```python
from build123d import *

# Parameters (mm, degrees)
SKETCH1_W   = 1.27
SKETCH1_H   = 25.4
SKETCH1_W_2 = 1.4732
SKETCH1_W_3 = 2.473987507
SKETCH1_H_2 = 76.2


with BuildPart() as part:
    # Sketch1 → Revolve1 (revolve)
    with BuildSketch(Plane.XY, mode=Mode.PRIVATE) as revolve1_sk:
        with Locations((23.675312493, 66.261527288)):
            Rectangle(SKETCH1_W, SKETCH1_H)
        Polygon((24.310312493, 53.561527288), (23.040312493, 53.561527288), (23.040312493, 28.161527288), (25.5143, 28.161527288), (25.5143, 53.561527288), align=None)
        with Locations((26.2509, 40.861527288)):
            Rectangle(SKETCH1_W_2, SKETCH1_H)
        with Locations((24.277306247, -9.938472712)):
            Rectangle(SKETCH1_W_3, SKETCH1_H_2)
    revolve(revolve1_sk.sketch.rotate(Axis((0, 0, 0), (0, 1, 0)), 90), axis=Axis((0, 0, 0), (0, 1, 0)))


solid = part.part
```
For this review, take the finished solid that the model builds, in its own axes (mm). A direction names the side the tool comes from. Give positions to 0.01 mm unless a question says otherwise; leave off trailing zeros. Loops run counter-clockwise (first coordinate to the right, second up) from the corner with the lowest first, then second, coordinate; pieces in that order, holes last. Notation, with made-up numbers: M 30.25,-29.75 L 36.25,-29.75 A24 cw 36.25,9.25 Z; hole C 11,52 d2. An arc over 180 degrees is marked long. One line per item, written item: value. Start each with the question number.
Q1. Add section B-B (z = 0). Give the boundary of the cut face in (x, y).
Q2. Clearance check with flat-ended pins moving along their axes: pin 1 Ø3 at (x, y) = (-5.5, 54.5) entering from -Z; pin 2 Ø1.5 at (y, z) = (-18.5, 9.5) entering from +X; pin 3 Ø8 at (x, y) = (17, 46.5) entering from +Z. State where each tip first meets the part, or that it passes through.
Q3. Add section A-A (x = 0). Give the boundary of the cut face in (y, z).
Q4. For L1, parallel to X at y = 65, z = 0; L2, parallel to X at y = -0.5, z = 0; L3, parallel to Z at x = 16, y = 24, list the stretches that pass through material, from the lowest coordinate up.
Q5. Add section C-C (y = -22.5). Give the boundary of the cut face in (x, z).
Q6. Draft analysis for pull direction X (two halves, no side actions). For faces 4 (the face through (-23, -48.038, -4)), 5 (the face through (14, 14.6, 18.3)), 6 (the face through (-18.24, 41.04, 19.89)), state which applies: released by +X, released by -X, zero draft, split by the parting line, or undercut.
Q7. Add section D-D (y = 49). Give the boundary of the cut face in (x, z) (1 decimal).
Q8. Machinability: for faces 1 (the face through (23.732, 66.439, 5.27)), 2 (the face through (10, 28.162, 24)), 3 (the face through (18, 78.962, -15)), which of the approach directions +Z, -Z, +X, -X, +Y, -Y give a long, thin tool a straight path to every point of the face, cutting with its end or side? Answer none if there is none.
Reply:
1. outline: M -26.99,28.16 L -25.51,28.16 L -25.51,-48.04 L -23.04,-48.04 L -23.04,78.96 L -24.31,78.96 L -24.31,53.56 L -26.99,53.56 Z; M 23.04,-48.04 L 25.51,-48.04 L 25.51,28.16 L 26.99,28.16 L 26.99,53.56 L 24.31,53.56 L 24.31,78.96 L 23.04,78.96 Z
2. pin 1: z = -26.64
2. pin 2: x = 23.97
2. pin 3: z = 23.65
3. outline: M -48.04,-25.51 L 28.16,-25.51 L 28.16,-26.99 L 53.56,-26.99 L 53.56,-24.31 L 78.96,-24.31 L 78.96,-23.04 L -48.04,-23.04 Z; M -48.04,23.04 L 78.96,23.04 L 78.96,24.31 L 53.56,24.31 L 53.56,26.99 L 28.16,26.99 L 28.16,25.51 L -48.04,25.51 Z
4. L1: -24.31 to -23.04, 23.04 to 24.31
4. L2: -25.51 to -23.04, 23.04 to 25.51
4. L3: -19.87 to -16.58, 16.58 to 19.87
5. outline: C 0,0 d51.03; hole C 0,0 d46.08
6. face 4: zero draft
6. face 5: undercut
6. face 6: split by the parting line
7. outline: C 0,0 d54; hole C 0,0 d46.1
8. face 1: +Y
8. face 2: -Y
8. face 3: +Z, -Z, +X, -X, +Y
